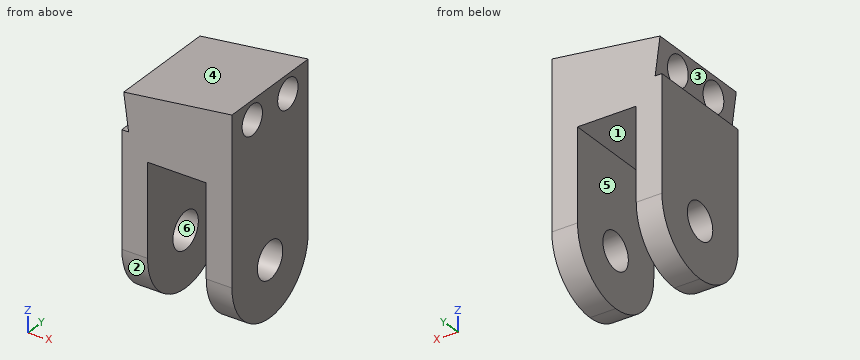
```python
from build123d import *

# Parameters (mm, degrees)
F0_W     = 15
F0_H     = 30
F1_DEPTH = 15
F2_W     = 8
F2_H     = 20
F3_DEPTH = 25.4
F4_R     = 7.49999
F5_R     = 2
F6_DEPTH = 25.4
F7_R     = 2.5
F8_DEPTH = 25.4


# Not quite as in the source:
# - a fillet or chamfer is up to 0.001 mm smaller than in the source, because OpenCascade refuses the exact size


with BuildPart() as f1:
    # F0 (on Front) → F1 (new body)
    with BuildSketch(Plane.XZ):
        Rectangle(F0_W, F0_H)
    extrude(amount=F1_DEPTH)

    # F2 (on face) → F3 (cut)
    with BuildSketch(Plane.XZ.offset(15)):
        with Locations((0, -5)):
            Rectangle(F2_W, F2_H)
        Polygon((-7.5, 15), (-7.5, 13), (-7.2379912664, 13.0349344978), align=None)
        Polygon((-7.2379912664, 13.0349344978), (-7.5, 13), (-7.5, 8.0614046952), (-6.5748539594, 8.0614046952), align=None)
        Polygon((-7.5, 15), (-7.2379912664, 13.0349344978), (7.5, 15), align=None)
    extrude(amount=-F3_DEPTH, mode=Mode.SUBTRACT)

    # F4 (radius 7.5 in the source; OpenCascade refuses exactly that, so slightly less here)
    f4_edges = [f1.edges().sort_by_distance(p)[0] for p in [
        (-5.75, -15, -15),
        (-5.75, 0, -15),
        (5.75, 0, -15),
        (5.75, -15, -15),
    ]]
    fillet(f4_edges, radius=F4_R)

    # F5 (on face) → F6 (cut)
    with BuildSketch(Plane(origin=(-5.403930131, 0, -0.7205240175), x_dir=(0, -1, 0), z_dir=(-0.9912279007, 0, -0.1321637201))):
        with Locations((4, 11.3289700367)):
            Circle(F5_R)
        with Locations((11, 11.3289700367)):
            Circle(F5_R)
    extrude(amount=-F6_DEPTH, mode=Mode.SUBTRACT)

    # F7 (on face) → F8 (cut)
    with BuildSketch(Plane(origin=(-7.5, 0, 0), x_dir=(0, -1, 0), z_dir=(-1, 0, 0))):
        with Locations((7.5, -7.5)):
            Circle(F7_R)
    extrude(amount=-F8_DEPTH, mode=Mode.SUBTRACT)


solid = f1.part
```
Verification items for the finished model (mm, model axes). Face numbers are marked on the shaded views. A direction names the side the tool comes from. Round coordinates to 2 decimals unless told otherwise and drop trailing zeros. Write each loop counter-clockwise with the first axis right and the second up, starting at its lowest first coordinate (ties: lowest second). Pieces come first, ordered by that corner, then holes. Notation, with made-up numbers: (48, 28) - (56, 28) arc R24 ccw to (56, 64) - close; hole circle Ø8 at (40.25, 81). An arc over 180 degrees is marked (long way). Answer as a JSON object with one key per item and string values. Group by question number.
Q1. Section check A-A, the plane z = 1.5. Enter the section's corners in (x, y).
Q2. Section check B-B, the plane y = -8. Enter the section's corners in (x, z), plus the area to 3 significant figures.
Q3. Go/stop test with flat-tipped pins: pin 1 Ø1.5 at (x, z) = (2.5, -5) entering from -Y; pin 2 Ø1 at (x, y) = (-0.5, -9.5) entering from +Z; pin 3 Ø4 at (x, y) = (-0.5, -11) entering from -Z; pin 4 Ø1.5 at (x, y) = (-3.5, -2.5) entering from -Z. Record where each tip stops, or that it passes through.
Q4. Mould release check, pull along Z, two halves, no side actions. Record for the marked faces 4, 5 and 6: released by +Z, released by -Z, zero draft, split by the parting line, or undercut.
Q5. Thickness scan on line 1 (X direction, y = -1.5, z = -7.25); line 2 (Z direction, x = -5.5, y = -5.75); line 3 (Z direction, x = 7.25, y = -9.75). Record the ranges inside material, lowest first.
Q6. Section check C-C, the plane y = -9.5. Enter the section's corners in (x, z), plus the area to 3 significant figures.
Q7. Section check D-D, the plane z = -8.25. Enter the section's corners in (x, y).
Q8. Tool access check on the marked faces 1, 2 and 3. Record the directions out of +Z, -Z, +X, -X, +Y, -Y that give a thin tool (end or side, any length) a straight path to the whole face; none if there is none.
Found:
{
 "1": {"outline": "(-7.5, -15) - (-4, -15) - (-4, 0) - (-7.5, 0) - close; (4, -15) - (7.5, -15) - (7.5, 0) - (4, 0) - close"},
 "2": {"outline": "(-7.5, -14.98) - (-4, -14.98) - (-4, -9.95) - (-7.5, -9.95) - close; (-7.5, -5.05) - (-4, -5.05) - (-4, 5) - (4, 5) - (4, -5.05) - (7.5, -5.05) - (7.5, 15) - (-7.24, 13.03) - (-6.57, 8.06) - (-7.5, 8.06) - close; (4, -14.98) - (7.5, -14.98) - (7.5, -9.95) - (4, -9.95) - close", "area": "238 mm^2"},
 "3": {"pin 1": "passes through", "pin 2": "stops at z = 14", "pin 3": "stops at z = 5", "pin 4": "stops at z = -13.54"},
 "4": {"face 4": "released by +Z", "face 5": "zero draft", "face 6": "undercut"},
 "5": {"line 1": "x = -7.5 to -4, 4 to 7.5", "line 2": "z = -14.79 to -9.29, -5.71 to 9.72, 11.67 to 13.27", "line 3": "z = -14.65 to -8.59, -6.41 to 10.82, 13.97 to 14.97"},
 "6": {"outline": "(-7.5, -14.73) - (-4, -14.73) - (-4, -9) - (-7.5, -9) - close; (-7.5, -6) - (-4, -6) - (-4, 5) - (4, 5) - (4, -6) - (7.5, -6) - (7.5, 11.09) - (-6.73, 9.2) - (-6.57, 8.06) - (-7.5, 8.06) - close; (-7.24, 13.03) - (-7.08, 11.82) - (7.5, 13.76) - (7.5, 15) - close; (4, -14.73) - (7.5, -14.73) - (7.5, -9) - (4, -9) - close", "area": "211 mm^2"},
 "7": {"outline": "(-7.5, -14.96) - (-4, -14.96) - (-4, -9.88) - (-7.5, -9.88) - close; (-7.5, -5.12) - (-4, -5.12) - (-4, -0.04) - (-7.5, -0.04) - close; (4, -14.96) - (7.5, -14.96) - (7.5, -9.88) - (4, -9.88) - close; (4, -5.12) - (7.5, -5.12) - (7.5, -0.04) - (4, -0.04) - close"},
 "8": {"face 1": "-Z, +Y, -Y", "face 2": "-Z, +X, -X, -Y", "face 3": "-X, +Y, -Y"}
}
